Geometry: see drawing. Coordinates: mm, zero at the bounding-box minimum. A direction names the side the tool comes from. Round coordinates to 2 decimals unless told otherwise and drop trailing zeros. Write each loop counter-clockwise with the first axis right and the second up, starting at its lowest first coordinate (ties: lowest second). Pieces come first, ordered by that corner, then holes. Notation, with made-up numbers: (-37, 46.5) -> (21, 46.5) arc R16 cw to (21, 63.5) -> close; hole circle Ø9 at (37.25, -9). An arc over 180 degrees is marked (long way). Use CSV: the item, a comma, the result in double quotes.
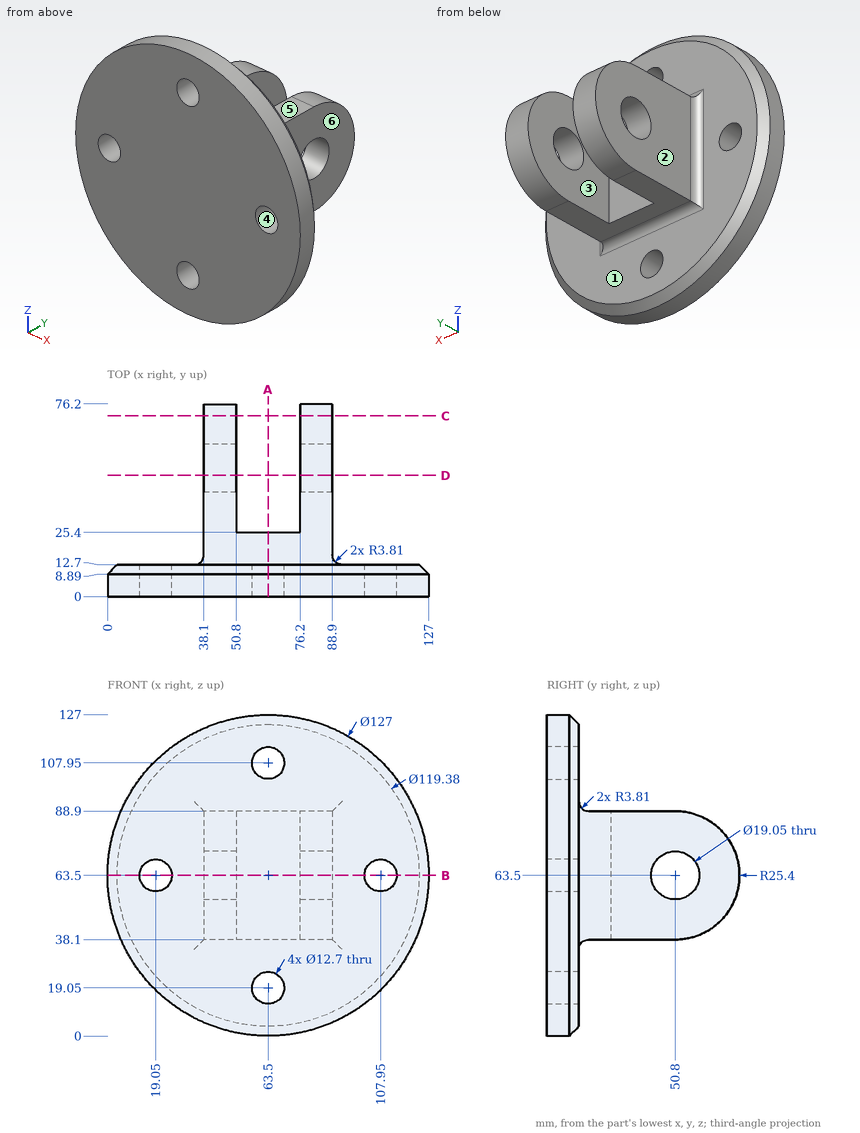
Item 1: First-contact query: pin 1 Ø10 at (y, z) = (19, 85) entering from -X; pin 2 Ø10.5 at (x, y) = (56, 29) entering from -Z; pin 3 Ø4 at (y, z) = (66.5, 53) entering from +X. Flat tips, straight axial feed; report the tip coordinate or a pass-through.
Worked answers:
pin 1,"stops at x = 37.16"
pin 2,"stops at z = 38.1"
pin 3,"stops at x = 88.9"
Item 2: Pull-direction query (X, two-part tool) for the marked faces 4, 5 and 6; classes: +X half, -X half, draft (parallel to the pull), parting line (faces both ways), or undercut.
Worked answers:
face 4,"undercut"
face 5,"draft"
face 6,"+X half"
Item 3: Section query D-D on y = 48. Return the cut outline in (x, z), plus the area to 3 significant figures.
Worked answers:
outline,"(38.1, 38.1) -> (50.8, 38.1) -> (50.8, 54.4) -> (38.1, 54.4) -> close; (38.1, 72.6) -> (50.8, 72.6) -> (50.8, 88.9) -> (38.1, 88.9) -> close; (76.2, 38.1) -> (88.9, 38.1) -> (88.9, 54.4) -> (76.2, 54.4) -> close; (76.2, 72.6) -> (88.9, 72.6) -> (88.9, 88.9) -> (76.2, 88.9) -> close"
area,"828 mm²"
Item 4: Section query B-B on z = 63.5. Give the number of separate pieces and of enclosed holes in the cut face, plus the area to 3 significant figures.
Worked answers:
separate pieces,"5"
enclosed holes,"0"
area,"2,730 mm²"
Item 5: Section query C-C on y = 71.5. Return the cut outline in (x, z), plus the area to 3 significant figures.
Worked answers:
outline,"(38.1, 48.78) -> (50.8, 48.78) -> (50.8, 78.22) -> (38.1, 78.22) -> close; (76.2, 48.78) -> (88.9, 48.78) -> (88.9, 78.22) -> (76.2, 78.22) -> close"
area,"748 mm²"
Item 6: Section query A-A on x = 63.5. Return the cut outline in (y, z).
Worked answers:
outline,"(0, 0) -> (8.89, 0) -> (12.7, 3.81) -> (12.7, 12.7) -> (0, 12.7) -> close; (0, 25.4) -> (12.7, 25.4) -> (12.7, 34.29) arc R3.81 cw to (16.51, 38.1) -> (25.4, 38.1) -> (25.4, 88.9) -> (16.51, 88.9) arc R3.81 cw to (12.7, 92.71) -> (12.7, 101.6) -> (0, 101.6) -> close; (0, 114.3) -> (12.7, 114.3) -> (12.7, 123.19) -> (8.89, 127) -> (0, 127) -> close"
Item 7: Line query: line 1 (X direction, y = 4.5, z = 63.5); line 2 (Y direction, x = 81, z = 63); line 3 (X direction, y = 61, z = 63.5). Output: solid intervals per line, ascending.
Worked answers:
line 1,"x = 0 to 12.7, 25.4 to 101.6, 114.3 to 127"
line 2,"y = 0 to 41.29, 60.31 to 76.2"
line 3,"x = 38.1 to 50.8, 76.2 to 88.9"
Item 8: Set-up query: the marked faces 1, 2 and 3. Return all of +Z, -Z, +X, -X, +Y, -Y with unobstructed straight access to the full face (end or side cutting, diameter ignored); none if empty.
Worked answers:
face 1,"+Y"
face 2,"+Z, -Z, -X, +Y"
face 3,"+Z, -Z, +Y"
